Design review of the part built by this model. Coordinates are the model's own, in mm. A direction names the side the tool comes from. Coordinates: 2 decimals unless noted, no trailing zeros. Loops run counter-clockwise (first coordinate to the right, second up) from the corner with the lowest first, then second, coordinate; pieces in that order, holes last. Notation, with made-up numbers: (24.25, 84.5) -> (64.25, 84.5) arc R16 cw to (64.25, 100.5) -> close; hole circle Ø2 at (28.5, 69). An arc over 180 degrees is marked (long way). Answer as a JSON object with one key per item and string values.
```python
from build123d import *

# Parameters (mm, degrees)
F0_W      = 225
F0_H      = 165
F1_DEPTH  = 30
F2_R      = 6.75
F3_DEPTH  = 15
F5_W      = 0.0118811131
F5_H      = 10.5422940105
F5_W_2    = 10.4881188869
F5_W_3    = 30
F5_H_2    = 7
F10_R     = 5.9
F11_DEPTH = 12.85
F12_DEPTH = 25
F15_W     = 8.7
F15_H     = 10
F15_W_2   = 40
F15_H_2   = 6
F17_R     = 5.05
F18_DEPTH = 10.6
F19_W     = 184.7800500691
F19_H     = 23.5
F20_DEPTH = 30
F21_W     = 169.1280193627
F21_H     = 10.5079561472
F22_DEPTH = 50


# Not quite as in the source:
# - a feature names something its author has since deleted; it is built from what else it names


with BuildPart() as f1:
    # F0 (on Top) → F1 (new body)
    with BuildSketch(Plane.XY):
        with Locations((112.5, 82.5)):
            Rectangle(F0_W, F0_H)
    extrude(amount=F1_DEPTH)

    # F2 (on face) → F3 (join)
    with BuildSketch(Plane.XY.offset(30)):
        with Locations((22, 127)):
            Circle(F2_R)
        with Locations((22, 92)):
            Circle(F2_R)
        with Locations((22, 57)):
            Circle(F2_R)
        with Locations((22, 22)):
            Circle(F2_R)
    extrude(amount=F3_DEPTH)

    # F5 (on face) → F6 (revolve, cut)
    with BuildSketch(Plane.XY.offset(30)):
        with Locations((43.9940594435, 16.1421531811)):
            Rectangle(F5_W, F5_H)
        with Locations((49.2440594435, 16.1421531811)):
            Rectangle(F5_W_2, F5_H)
        Polygon((58.2381188869, 21.4133001864), (54.4881188869, 21.4133001864), (54.4881188869, 10.8710061759), (54.4881188869, 8.0633001864), (58.2381188869, 8.0633001864), (58.2381188869, 14.4133001864), align=None)
        with Locations((73.2381188869, 17.9133001864)):
            Rectangle(F5_W_3, F5_H_2)
    revolve(axis=Axis((49.2381188869, 21.4133001864, 30), (1, 0, 0)), mode=Mode.SUBTRACT)

    # F7 (on face) → F8 (revolve, cut)
    with BuildSketch(Plane.XY.offset(30)):
        Polygon((44, 57), (44, 46.25), (54.5, 46.25), (54.5, 43.65), (58.25, 43.65), (58.25, 50), (88.25, 50), (88.25, 57), (58.25, 57), (54.5, 57), align=None)
    revolve(axis=Axis((49.25, 57, 30), (1, 0, 0)), mode=Mode.SUBTRACT)

    # F10 (on face) → F11 (join)
    with BuildSketch(Plane.XY.offset(30)):
        with Locations((62.1212087572, 121.5757578611)):
            Circle(F10_R)
        with Locations((62.1212087572, 91.7575731874)):
            Circle(F10_R)
    extrude(amount=F11_DEPTH)

    # F10 (on face) → F12 (join)
    with BuildSketch(Plane.XY.offset(30)):
        with Locations((62.1212087572, 121.5757578611)):
            Circle(F10_R)
        with Locations((62.1212087572, 91.7575731874)):
            Circle(F10_R)
        with Locations((96.6326966882, 92.5912261009)):
            Circle(F10_R)
        with Locations((96.1869060993, 121.1215853691)):
            Circle(F10_R)
        with Locations((114.9099543691, 22.1569109708)):
            Circle(F10_R)
        with Locations((129.1751265526, 121.1215853691)):
            Circle(F10_R)
        with Locations((130.0667077303, 92.5912261009)):
            Circle(F10_R)
        with Locations((114.4641637802, 57.3740676045)):
            Circle(F10_R)
    extrude(amount=F12_DEPTH)

    # F13 (on face) → F14 (revolve, cut)
    with BuildSketch(Plane.XY.offset(30)):
        Polygon((160.9424221039, 28.7878794968), (152.2424221039, 28.7878794968), (152.2424221039, 18.7878794968), (160.9424221039, 18.7878794968), (160.9424221039, 15.7878794968), (164.6924221039, 15.7878794968), (164.6924221039, 22.7878794968), (204.6924221039, 22.7878794968), (204.6924221039, 28.7878794968), (164.6924221039, 28.7878794968), align=None)
    revolve(axis=Axis((184.6924221039, 28.7878794968, 30), (1, 0, 0)), mode=Mode.SUBTRACT)

    # F15 (on face) → F16 (revolve, cut)
    with BuildSketch(Plane.XY.offset(30)):
        with Locations((156.6197043896, 69.1212128103)):
            Rectangle(F15_W, F15_H)
        Polygon((164.7197043896, 74.1212128103), (160.9697043896, 74.1212128103), (160.9697043896, 64.1212128103), (160.9697043896, 61.1212128103), (164.7197043896, 61.1212128103), (164.7197043896, 68.1212128103), align=None)
        with Locations((184.7197043896, 71.1212128103)):
            Rectangle(F15_W_2, F15_H_2)
    revolve(axis=Axis((184.7197043896, 74.1212128103, 30), (1, 0, 0)), mode=Mode.SUBTRACT)

    # F17 (on face) → F18 (join)
    with BuildSketch(Plane.XY.offset(30)):
        with Locations((162.1633470058, 113.5432049632)):
            Circle(F17_R)
        with Locations((199.1636604071, 114.4347786903)):
            Circle(F17_R)
    extrude(amount=F18_DEPTH)

    # F19 (on face) → F20 (join)
    with BuildSketch(Plane.XY.offset(30)):
        with Locations((132.609969005, 153.3750020266)):
            Rectangle(F19_W, F19_H)
    extrude(amount=F20_DEPTH)

    # F21 (on face) → F22 (cut)
    with BuildSketch(Plane.XY.offset(60)):
        with Locations((134.2664714903, 154.7421440482)):
            Rectangle(F21_W, F21_H)
    extrude(amount=-F22_DEPTH, mode=Mode.SUBTRACT)


solid = f1.part
```
1) Wall thickness on probe 1 along Y at (x, z) = (86.5, 54) (3 decimals); probe 2 along Y at (x, z) = (58.5, 53) (3 decimals); probe 3 along X at (y, z) = (157, 39.5): over which ranges is each line inside the solid? List them lowest first.
Completed:
{"probe 1": "141.625 to 149.488, 159.996 to 165.125", "probe 2": "87.1 to 96.416, 116.918 to 126.234, 141.625 to 149.488, 159.996 to 165.125", "probe 3": "40.22 to 49.7, 218.83 to 225"}
2) Clearance check with flat-ended pins moving along their axes: pin 1 Ø13 at (x, y) = (95.5, 119.5) entering from +Z; pin 2 Ø2 at (x, y) = (152, 27) entering from +Z; pin 3 Ø1 at (y, z) = (52, 48.5) entering from -X. State where each tip first meets the part, or that it passes through.
Completed:
{"pin 1": "z = 55", "pin 2": "z = 30", "pin 3": "x = 111.14"}
3) Add section C-C, the plane x = 191.5. Give the boundary of the cut face in (y, z) (3 decimals), and give its area (3 significant figures).
Completed:
{"outline": "(0, 0) -> (165, 0) -> (165, 30) -> (165.125, 30) -> (165.125, 60) -> (159.996, 60) -> (159.996, 10) -> (149.488, 10) -> (149.488, 60) -> (141.625, 60) -> (141.625, 30) -> (80.121, 30) arc R6 cw to (68.121, 30) -> (34.788, 30) arc R6 cw to (22.788, 30) -> (0, 30) -> close", "area": "5,020 mm²"}
4) Add section A-A, the plane x = 149.5. Give the boundary of the cut face in (y, z) (3 decimals).
Completed:
{"outline": "(0, 0) -> (165, 0) -> (165, 30) -> (165.125, 30) -> (165.125, 60) -> (159.996, 60) -> (159.996, 10) -> (149.488, 10) -> (149.488, 60) -> (141.625, 60) -> (141.625, 30) -> (0, 30) -> close"}
5) For faces 4 (the cylindrical face through (56.401, 56.706, 16.653)), 5 (the flat face through (162, 114, 40.6)), 6 (the flat face through (96, 121, 55)), list the 3-axis set-ups (+Z, -Z, +X, -X, +Y, -Y) from which the entire face can be reached by the end or side of a thin tool; tool diameter is ignored.
Completed:
{"face 4": "+Z", "face 5": "+Z, +X, -Y", "face 6": "+Z, +X, -X, -Y"}
6) Add section D-D, the plane y = 75.5. Give the boundary of the cut face in (x, z).
Completed:
{"outline": "(0, 0) -> (225, 0) -> (225, 30) -> (204.72, 30) -> (204.72, 24.16) -> (164.72, 24.16) -> (164.72, 17.07) -> (160.97, 17.07) -> (160.97, 20.1) -> (152.27, 20.1) -> (152.27, 30) -> (0, 30) -> close"}
7) The part is to be moulded in two halves that separate along X. For faces 1 (the flat face through (111, 84, 0)), 2 (the flat face through (225, 153, 45)), 3 (the cylindrical face through (157, 74, 20)), say which applies: pulls with the +X half, pulls with the -X half, needs draft (parallel to the pull), parting line crosses it, or undercut.
Completed:
{"face 1": "needs draft", "face 2": "pulls with the +X half", "face 3": "undercut"}
